Part print with two shaded views. Sizes in mm from the minimum x, y, z corner. A direction names the side the tool comes from. Round coordinates to 2 decimals unless told otherwise and drop trailing zeros. Order: outer loops, then holes, each group sorted by start corner. A loop starts at its lowest first (then second) coordinate and runs counter-clockwise, first axis right, second up. Notation, with made-up numbers: M -7.75,31.25 L 44.25,31.25 A31 cw 44.25,64.25 Z; hole C -10,59.25 d7. An arc over 180 degrees is marked long. One line per question, with ' | ' between items.
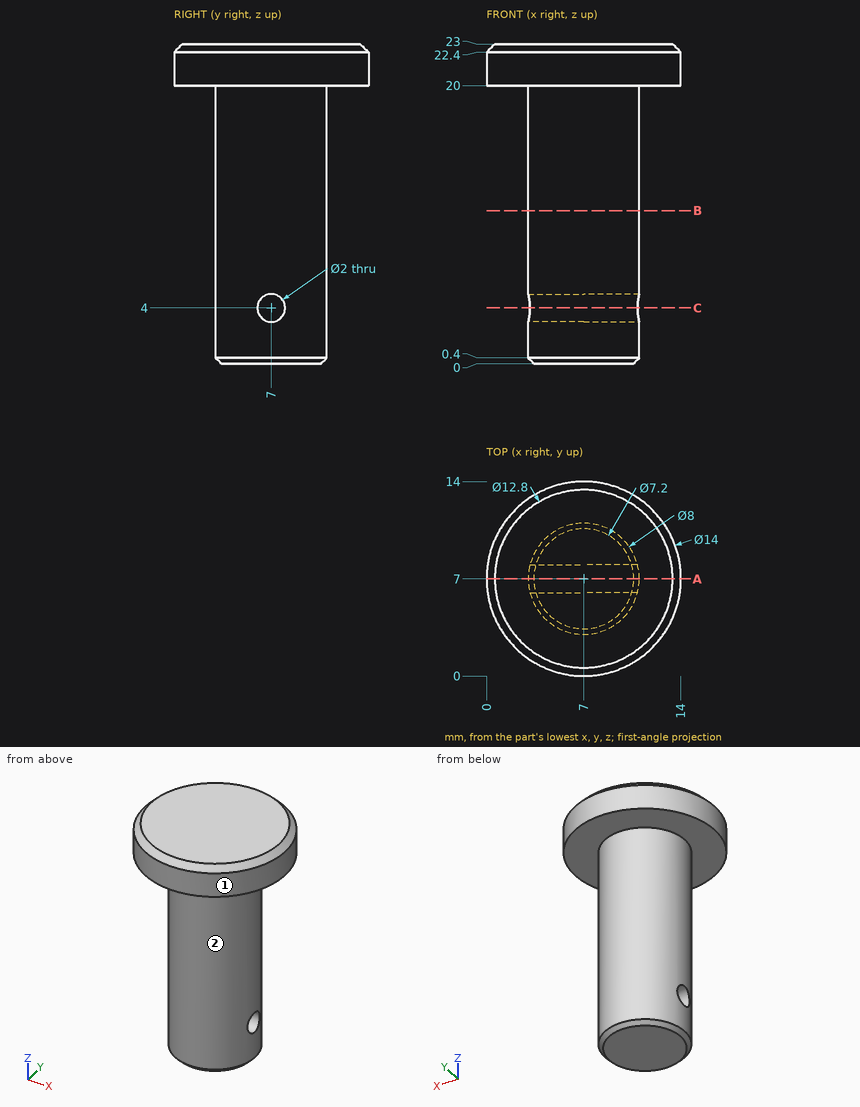
1) Probe line 1 (Z direction, x = 8.75, y = 7); line 2 (Y direction, x = 5.25, z = 4); line 3 (Z direction, x = 1.75, y = 4). List the from-to ranges inside material, lowest first. Write a range as [from, to].
The answers:
line 1: z = [0, 3], [5, 23] | line 2: y = [3.4, 6], [8, 10.6] | line 3: z = [20, 23]
2) Saw through at A-A (y = 7). List the corners of the cut face in (x, z).
The answers:
outline: M 0,20 L 3,20 L 3,5 L 11,5 L 11,20 L 14,20 L 14,22.4 L 13.4,23 L 0.6,23 L 0,22.4 Z; M 3,0.4 L 3.4,0 L 10.6,0 L 11,0.4 L 11,3 L 3,3 Z
3) Saw through at B-B (z = 11). List the corners of the cut face in (x, y), plus the area to 3 significant figures.
The answers:
outline: C 7,7 d8 | area: 50.3 mm²
4) Which spindle directions (+Z, -Z, +X, -X, +Y, -Y) get a long thin tool onto all of the face, cutting with end or side? Do the marked faces 1 and 2. Say none if no direction does.
The answers:
face 1: +Z, -Z | face 2: -Z
5) Saw through at C-C (z = 4). List the corners of the cut face in (x, y).
The answers:
outline: M 3.13,6 A4 ccw 10.87,6 Z; M 3.13,8 L 10.87,8 A4 ccw Z
6) Drop flat-ended pins along their axis: pin 1 (3 mm diameter, centred on y = 2.5, z = 18, fed in from -X); pin 2 (2.5 mm diameter, centred on y = 7, z = 4, fed in from -X); pin 3 (3 mm diameter, centred on y = 7, z = 4, fed in from +X). Give the stop position or say it passes through.
The answers:
pin 1: stops at x = 4.35 | pin 2: stops at x = 3 | pin 3: stops at x = 11
